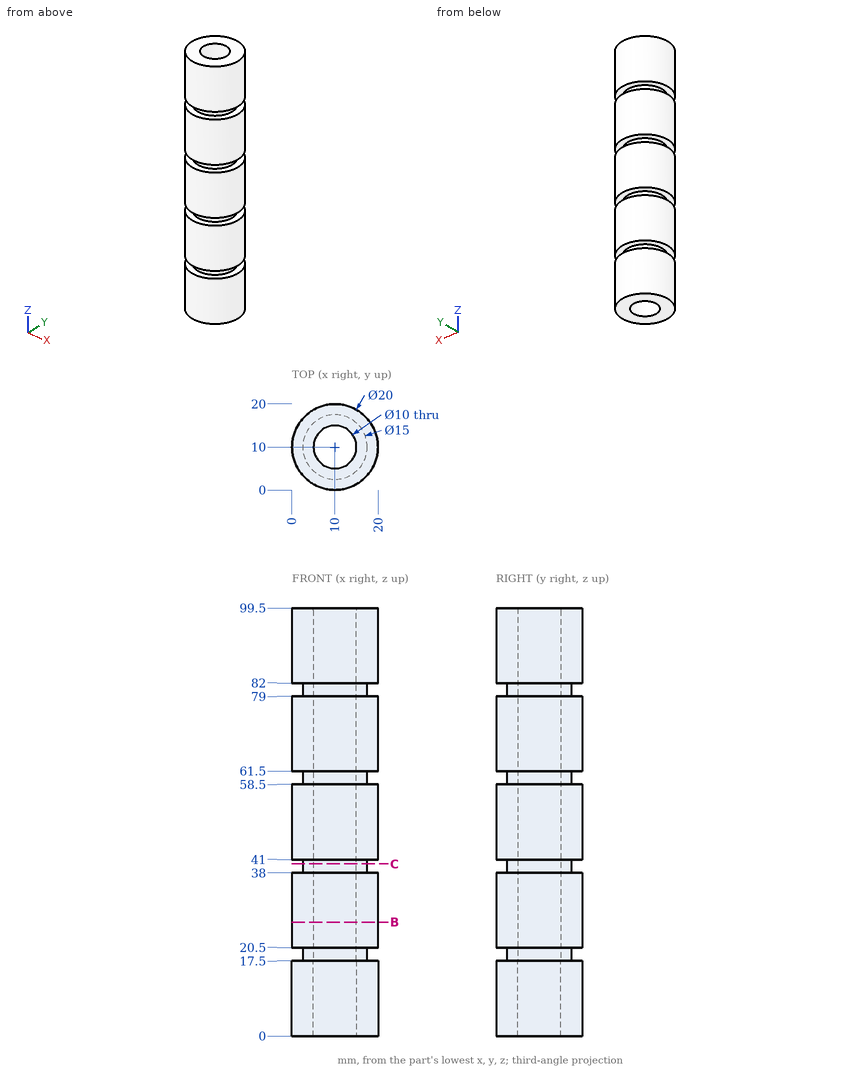
Design review of the part shown in the three views and the two pictorial views. Dimensions are in mm from the part's minimum x, y and z. Round coordinates to 2 decimals unless told otherwise and drop trailing zeros. Loops run counter-clockwise (first coordinate to the right, second up) from the corner with the lowest first, then second, coordinate; pieces in that order, holes last. Notation, with made-up numbers: M 43.25,39 L 49.25,39 A4 ccw 49.25,46 Z; hole C 68,-33.75 d10. An arc over 180 degrees is marked long. Answer as a JSON object with one key per item and string values.
Item 1: We need section C-C on z = 40. Give the boundary of the cut face in (x, y), and give its area (3 significant figures).
Answer sheet:
{"outline": "C 10,10 d15; hole C 10,10 d10", "area": "98.2 mm^2"}
Item 2: Clearance check with flat-ended pins moving along their axes: P1, Ø8, axis at y = 2.5, z = 58.5, coming from the +X side; P2, Ø4, axis at x = 2.5, z = 44.5, coming from the +Y side; P3, Ø8, axis at x = 12, z = 55.5, coming from the +Y side; P4, Ø1.5, axis at x = 5.5, z = 47.5, coming from the -Y side. State where each tip first meets the part, or that it passes through.
Answer sheet:
{"P1": "stops at x = 19.37", "P2": "stops at y = 18.35", "P3": "stops at y = 20", "P4": "stops at y = 0.73"}
Item 3: Wall thickness on L1, parallel to Z at x = 18, y = 14.5; L2, parallel to Y at x = 10, z = 4; L3, parallel to Y at x = 7, z = 6.5: over which ranges is each line inside the solid? List them lowest first. Write a range as from..to.
Answer sheet:
{"L1": "z = 0..17.5, 20.5..38, 41..58.5, 61.5..79, 82..99.5", "L2": "y = 0..5, 15..20", "L3": "y = 0.46..6, 14..19.54"}
Item 4: We need section B-B on z = 26.5. Give the boundary of the cut face in (x, y).
Answer sheet:
{"outline": "C 10,10 d20; hole C 10,10 d10"}
